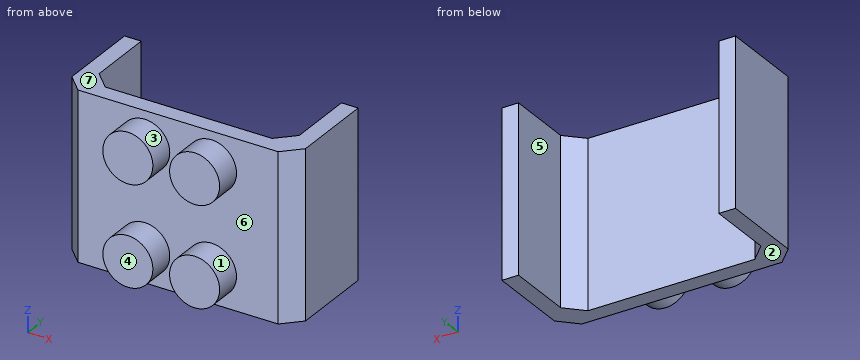
from build123d import *

# Parameters (mm, degrees)
F1_DEPTH = 50
F2_SIZE  = 5
F3_R     = 7.5
F4_DEPTH = 8


with BuildPart() as f1:
    # F0 (on Top) → F1 (new body)
    with BuildSketch(Plane.XY):
        Polygon((-30, 19), (-35, 19), (-35, -11), (0, -11), (35, -11), (35, 19), (30, 19), (30, -6), (0, -6), (-30, -6), align=None)
    extrude(amount=F1_DEPTH)

    # F2
    f2_edges = [f1.edges().sort_by_distance(p)[0] for p in [
        (-30, -6, 25),
        (30, -6, 25),
        (-35, -11, 25),
        (35, -11, 25),
    ]]
    chamfer(f2_edges, length=F2_SIZE)

    # F3 (on face) → F4 (join)
    with BuildSketch(Plane.XZ.offset(11)):
        with Locations((-10, 40)):
            Circle(F3_R)
        with Locations((-10, 10)):
            Circle(F3_R)
        with Locations((10, 40)):
            Circle(F3_R)
        with Locations((10, 10)):
            Circle(F3_R)
    extrude(amount=F4_DEPTH)


solid = f1.part
Part model, mm, in its own coordinate system. Face numbers are marked on the shaded views. A direction names the side the tool comes from. Coordinates: 2 decimals unless noted, no trailing zeros. Write each loop counter-clockwise with the first axis right and the second up, starting at its lowest first coordinate (ties: lowest second). Pieces come first, ordered by that corner, then holes. Notation, with made-up numbers: (35.25, 65) - (39.25, 65) arc R30 ccw to (39.25, 97) - close; hole circle Ø1 at (-10, -38). An arc over 180 degrees is marked (long way). Put each result on its own line as item: value.
1. Flat gauge pin, fed straight in: pin 1 Ø6 at (x, z) = (16, 33.5) entering from +Y. Where does the tip first touch, or does it go through?
Final values:
pin 1: stops at y = -6
2. Two-plate mould, pull along Z, no slides. Class the marked faces 1, 2, 3 and 4: +Z half, -Z half, draft (parallel to the pull), parting line (faces both ways), or undercut.
Final values:
face 1: undercut
face 2: -Z half
face 3: undercut
face 4: draft
3. Probe line 1 along X through (y, z) = (1.5, 18); line 2 along Y through (x, z) = (-11.5, 32.5); line 3 along Z through (x, y) = (-10.5, -13). List the from-to ranges inside material, lowest first. Write a range as [from, to].
Final values:
line 1: x = [-35, -30], [30, 35]
line 2: y = [-11, -6]
line 3: z = [2.52, 17.48], [32.52, 47.48]
4. 3-axis set-ups, long thin cutter, end or side, ignore diameter. For the marked faces 5, 6 and 7: which of +Z, -Z, +X, -X, +Y, -Y reach the whole face in a straight line?
Final values:
face 5: +Z, -Z, +Y
face 6: -Y
face 7: +Z, +X, -X, +Y, -Y
5. Band-saw the part on D-D (z = 40). Write the cut outline in (x, y).
Final values:
outline: (-35, -6) - (-30, -11) - (-17.5, -11) - (-17.5, -19) - (-2.5, -19) - (-2.5, -11) - (2.5, -11) - (2.5, -19) - (17.5, -19) - (17.5, -11) - (30, -11) - (35, -6) - (35, 19) - (30, 19) - (30, -1) - (25, -6) - (-25, -6) - (-30, -1) - (-30, 19) - (-35, 19) - close
6. Band-saw the part on A-A (y = 14). Write the cut outline in (x, z), then the cut area to 3 significant figures.
Final values:
outline: (-35, 0) - (-30, 0) - (-30, 50) - (-35, 50) - close; (30, 0) - (35, 0) - (35, 50) - (30, 50) - close
area: 500 mm²
7. Band-saw the part on C-C (x = -16). Write the cut outline in (y, z), then the cut area to 3 significant figures.
Final values:
outline: (-19, 5.5) - (-11, 5.5) - (-11, 0) - (-6, 0) - (-6, 50) - (-11, 50) - (-11, 44.5) - (-19, 44.5) - (-19, 35.5) - (-11, 35.5) - (-11, 14.5) - (-19, 14.5) - close
area: 394 mm²
8. Band-saw the part on B-B (z = 27.5). Write the cut outline in (x, y), then the cut area to 3 significant figures.
Final values:
outline: (-35, -6) - (-30, -11) - (30, -11) - (35, -6) - (35, 19) - (30, 19) - (30, -1) - (25, -6) - (-25, -6) - (-30, -1) - (-30, 19) - (-35, 19) - close
area: 600 mm²
